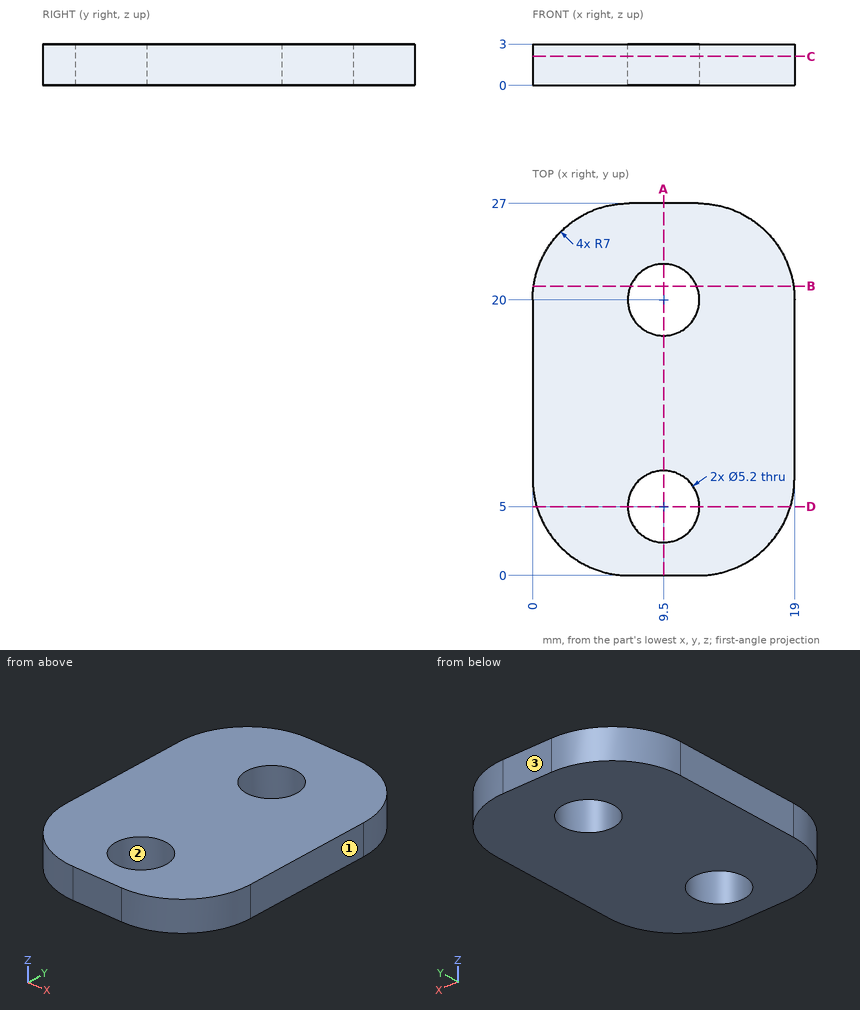
Can you work these out from the drawing? Everything is in mm from the part's minimum corner. Coordinates: 2 decimals unless noted, no trailing zeros. Loops run counter-clockwise (first coordinate to the right, second up) from the corner with the lowest first, then second, coordinate; pieces in that order, holes last.
1) Imagine slicing it at A-A (x = 9.5). List the corners of the cut face in (y, z) for me.
Reported:
outline: (0, 0) - (2.4, 0) - (2.4, 3) - (0, 3) - close; (7.6, 0) - (17.4, 0) - (17.4, 3) - (7.6, 3) - close; (22.6, 0) - (27, 0) - (27, 3) - (22.6, 3) - close
2) Thinking about a two-plate mould opening in Y: for the marked faces 1, 2 and 3, which applies, released by +Y, released by -Y, zero draft, split by the parting line, or undercut?
Reported:
face 1: zero draft
face 2: undercut
face 3: released by +Y
3) Please list where these lines run through material, in increasing order: line 1 along Y through (x, z) = (9.5, 1.3); line 2 along Y through (x, z) = (7.75, 1.25); line 3 along X through (y, z) = (21, 2.1).
Reported:
line 1: y = 0 to 2.4, 7.6 to 17.4, 22.6 to 27
line 2: y = 0 to 3.08, 6.92 to 18.08, 21.92 to 27
line 3: x = 0.07 to 7.1, 11.9 to 18.93
4) Imagine slicing it at D-D (y = 5). List the corners of the cut face in (x, z) for me.
Reported:
outline: (0.29, 0) - (6.9, 0) - (6.9, 3) - (0.29, 3) - close; (12.1, 0) - (18.71, 0) - (18.71, 3) - (12.1, 3) - close
5) Will this pin go through, and if not, where does the flat tip stop? pin 1 Ø1 at (x, z) = (16, 1) entering from -Y.
Reported:
pin 1: stops at y = 0.94
6) Imagine slicing it at C-C (z = 2.1). List the corners of the cut face in (x, y) for me, and give its area (3 significant figures).
Reported:
outline: (0, 7) arc R7 ccw to (7, 0) - (12, 0) arc R7 ccw to (19, 7) - (19, 20) arc R7 ccw to (12, 27) - (7, 27) arc R7 ccw to (0, 20) - close; hole circle Ø5.2 at (9.5, 5); hole circle Ø5.2 at (9.5, 20)
area: 428 mm2
7) Imagine slicing it at B-B (y = 21). List the corners of the cut face in (x, z) for me.
Reported:
outline: (0.07, 0) - (7.1, 0) - (7.1, 3) - (0.07, 3) - close; (11.9, 0) - (18.93, 0) - (18.93, 3) - (11.9, 3) - close
